```python
from build123d import *

# Parameters (mm, degrees)
RESSALTO_EXTRUS_O1_DEPTH = 4
FILETE1_R                = 3
M3_CLEARANCE_HOLE1_D     = 3.2
FURO_COM_FOLGA_DE_M32_D  = 2.87
M3_CLEARANCE_HOLE2_D     = 3.2
SKETCH3_W                = 27.430623534
SKETCH3_H                = 190
CUT_EXTRUDE1_DEPTH       = 10
BOSS_EXTRUDE1_DEPTH      = 4
FILLET3_R                = 3
BOSS_EXTRUDE3_DEPTH      = 4
M3_CLEARANCE_HOLE4_D     = 3.2
FILLET5_R                = 3
M5_CLEARANCE_HOLE1_D     = 5.3
SKETCH15_R               = 3
CUT_EXTRUDE6_DEPTH       = 5
SKETCH17_W               = 196
SKETCH17_H               = 23.942856981
CUT_EXTRUDE8_DEPTH       = 5
M3_CLEARANCE_HOLE6_D     = 3.2
M3_CLEARANCE_HOLE5_D     = 3.2
CUT_EXTRUDE9_DEPTH       = 4


with BuildPart() as part:
    # Esboço1 → Ressalto-extrusão1 (new body)
    with BuildSketch(Plane.XY):
        with BuildLine():
            Line((168.243612151, -138.115636704), (-79.756387849, -138.115636704))
            ThreePointArc((-79.756387849, -138.115636704), (-80.46349463, -137.822743485), (-80.756387849, -137.115636704))
            Line((-80.756387849, -137.115636704), (-80.756387849, 48.884363296))
            ThreePointArc((-80.756387849, 48.884363296), (-79.877708192, 51.005683639), (-77.756387849, 51.884363296))
            Line((-77.756387849, 51.884363296), (166.243612151, 51.884363296))
            ThreePointArc((166.243612151, 51.884363296), (168.364932495, 51.005683639), (169.243612151, 48.884363296))
            Line((169.243612151, 48.884363296), (169.243612151, -137.115636704))
            ThreePointArc((169.243612151, -137.115636704), (168.950718933, -137.822743485), (168.243612151, -138.115636704))
        make_face()
        with BuildLine():
            Line((-36.756387849, -93.115636704), (-55.756387849, -93.115636704))
            Line((-55.756387849, -93.115636704), (-55.756387849, -79.115636704))
            Line((-55.756387849, -79.115636704), (-55.756387849, 27.884363296))
            ThreePointArc((-55.756387849, 27.884363296), (-54.877708192, 30.005683639), (-52.756387849, 30.884363296))
            Line((-52.756387849, 30.884363296), (141.243612151, 30.884363296))
            ThreePointArc((141.243612151, 30.884363296), (143.364932495, 30.005683639), (144.243612151, 27.884363296))
            Line((144.243612151, 27.884363296), (144.243612151, -79.115636704))
            Line((144.243612151, -79.115636704), (144.243612151, -93.115636704))
            Line((144.243612151, -93.115636704), (125.243612151, -93.115636704))
            Line((125.243612151, -93.115636704), (125.243612151, -107.115636704))
            ThreePointArc((125.243612151, -107.115636704), (124.950718933, -107.822743485), (124.243612151, -108.115636704))
            Line((124.243612151, -108.115636704), (-35.756387849, -108.115636704))
            ThreePointArc((-35.756387849, -108.115636704), (-36.46349463, -107.822743485), (-36.756387849, -107.115636704))
            Line((-36.756387849, -107.115636704), (-36.756387849, -93.115636704))
        make_face(mode=Mode.SUBTRACT)
    extrude(amount=RESSALTO_EXTRUS_O1_DEPTH)

    # Filete1
    filete1_edges = [part.edges().sort_by_distance(p)[0] for p in [
        (-55.756387849, -93.115636704, 2),
        (-36.756387849, -93.115636704, 2),
        (125.243612151, -93.115636704, 2),
        (144.243612151, -93.115636704, 2),
    ]]
    fillet(filete1_edges, radius=FILETE1_R)

    # M3 Clearance Hole1 (through all)
    with Locations(Plane(origin=(0, 0, 0), x_dir=(-1, 0, 0), z_dir=(0, 0, -1))):
        with Locations((-164.230041881, -97.102981335), (43.669958119, -97.102981335), (75.742817578, -97.102981335)):
            Hole(M3_CLEARANCE_HOLE1_D / 2)

    # Furo com folga de M32 (through all)
    with Locations(Plane.XY.offset(4)):
        with Locations((44.243612151, 46.98714614)):
            Hole(FURO_COM_FOLGA_DE_M32_D / 2)

    # M3 Clearance Hole2 (through all)
    with Locations(Plane.XY.offset(4)):
        with Locations((161.560317261, 35.480164232), (161.560317261, 4.480164232)):
            Hole(M3_CLEARANCE_HOLE2_D / 2)

    # Sketch3 → Cut-Extrude1 (cut)
    with BuildSketch(Plane.XY.offset(4)):
        with Locations((169.958923918, -43.115636704)):
            Rectangle(SKETCH3_W, SKETCH3_H)
    extrude(amount=-CUT_EXTRUDE1_DEPTH, mode=Mode.SUBTRACT)

    # Sketch5 → Boss-Extrude1 (add)
    with BuildSketch(Plane(origin=(0, 0, 0), x_dir=(-1, 0, 0), z_dir=(0, 0, -1))):
        with BuildLine():
            Line((-145.240285588, -97.500155699), (-140.243612151, -97.500155699))
            Line((-140.243612151, -97.500155699), (-140.243612151, 27.941506315))
            ThreePointArc((-140.243612151, 27.941506315), (-139.345176524, 30.025791447), (-137.244156422, 30.884363296))
            Line((-137.244156422, 30.884363296), (-145.240285588, 30.884363296))
            Line((-145.240285588, 30.884363296), (-145.240285588, -97.500155699))
        make_face()
    extrude(amount=-BOSS_EXTRUDE1_DEPTH)

    # Fillet3
    fillet3_edges = [part.edges().sort_by_distance(p)[0] for p in [
        (156.243612151, 51.884363296, 2),
    ]]
    fillet(fillet3_edges, radius=FILLET3_R)

    # Sketch10 → Boss-Extrude3 (add)
    with BuildSketch(Plane(origin=(0, 0, 0), x_dir=(-1, 0, 0), z_dir=(0, 0, -1))):
        with BuildLine():
            Line((-156.243612151, -138.115636704), (-156.243612151, 48.884363296))
            ThreePointArc((-156.243612151, 48.884363296), (-155.364932495, 51.005683639), (-153.243612151, 51.884363296))
            Line((-153.243612151, 51.884363296), (-163.743612151, 51.884363296))
            Line((-163.743612151, 51.884363296), (-163.743612151, -138.115636704))
            Line((-163.743612151, -138.115636704), (-156.243612151, -138.115636704))
        make_face()
    extrude(amount=-BOSS_EXTRUDE3_DEPTH)

    # M3 Clearance Hole4 (through all)
    with Locations(Plane(origin=(0, 0, 0), x_dir=(-1, 0, 0), z_dir=(0, 0, -1))):
        with Locations((-160.743612151, -101.615636704), (-160.743612151, -132.615636704), (-129.743612151, -132.615636704), (-129.743612151, -101.615636704)):
            Hole(M3_CLEARANCE_HOLE4_D / 2)

    # Fillet5
    fillet5_edges = [part.edges().sort_by_distance(p)[0] for p in [
        (140.243612151, -93.115636704, 2),
        (163.743612151, 51.884363296, 2),
    ]]
    fillet(fillet5_edges, radius=FILLET5_R)

    # M5 Clearance Hole1 (through all)
    with Locations(Plane(origin=(0, 0, 0), x_dir=(-1, 0, 0), z_dir=(0, 0, -1))):
        with Locations((-115.03361215, -125.8856367), (26.54638785, -125.8856367), (-44.189907873, -129.865636704)):
            Hole(M5_CLEARANCE_HOLE1_D / 2)

    # Sketch15 → Cut-Extrude6 (cut, through all)
    with BuildSketch(Plane(origin=(0, 0, 0), x_dir=(-1, 0, 0), z_dir=(0, 0, -1))):
        with Locations((-145.243612151, -117.115636704)):
            Circle(SKETCH15_R)
    extrude(amount=-CUT_EXTRUDE6_DEPTH, mode=Mode.SUBTRACT)

    # Sketch17 → Cut-Extrude8 (cut)
    with BuildSketch(Plane(origin=(0, 0, 0), x_dir=(-1, 0, 0), z_dir=(0, 0, -1))):
        with Locations((-42.243612151, 39.912934806)):
            Rectangle(SKETCH17_W, SKETCH17_H)
    extrude(amount=-CUT_EXTRUDE8_DEPTH, mode=Mode.SUBTRACT)

    # M3 Clearance Hole6 (through all)
    with Locations(Plane(origin=(0, 0, 0), x_dir=(-1, 0, 0), z_dir=(0, 0, -1))):
        with Locations((-148.743612151, -78.347886704), (-148.743612151, -18.347886704), (-148.743612151, 41.652113296), (60.256387849, 41.652113296), (60.256387849, -18.347886704), (60.256387849, -78.347886704), (72.959751747, -51.945636704)):
            Hole(M3_CLEARANCE_HOLE6_D / 2)

    # M3 Clearance Hole5 (through all)
    with Locations(Plane.XY.offset(4)):
        with Locations((-75.756387849, 41.652113296), (-75.756387849, 48.152113296), (158.743612151, 48.152113296), (158.743612151, 41.652113296)):
            Hole(M3_CLEARANCE_HOLE5_D / 2)

    # Sketch22 → Cut-Extrude9 (cut)
    with BuildSketch(Plane(origin=(0, 0, 0), x_dir=(-1, 0, 0), z_dir=(0, 0, -1))):
        with BuildLine():
            Line((-46.840844325, -129.865636704), (-46.840844325, -123.2156367))
            ThreePointArc((-46.840844325, -123.2156367), (-44.189907873, -120.564700249), (-41.538971422, -123.2156367))
            Line((-41.538971422, -123.2156367), (-41.538971422, -129.865636704))
            ThreePointArc((-41.538971422, -129.865636704), (-44.189907873, -132.516573155), (-46.840844325, -129.865636704))
        make_face()
    extrude(amount=-CUT_EXTRUDE9_DEPTH, mode=Mode.SUBTRACT)


solid = part.part
```
Could you check a few things on this model? Use its own coordinates, in mm. Give positions to 0.01 mm unless a question says otherwise; leave off trailing zeros. Write each loop counter-clockwise with the first axis right and the second up, starting at its lowest first coordinate (ties: lowest second). Pieces come first, ordered by that corner, then holes. Notation, with made-up numbers: (-24, 64.5) -> (-6, 64.5) arc R24 ccw to (-6, 95.5) -> close; hole circle Ø5 at (86, -1.5). An arc over 180 degrees is marked (long way). Write each question's results on one line, items separated by ' | '.
1. I want a section at C-C, the plane x = 50. Write out the boundary of the cut face in (y, z).
Check sheet entries:
outline: (-138.12, 0) -> (-108.12, 0) -> (-108.12, 4) -> (-138.12, 4) -> close
2. Will these pins go through, and if not, where does the flat tip stop? pin 1 Ø1 at (x, z) = (44, 3) entering from +Y; pin 2 Ø1.9 at (x, y) = (129.74, -132.62) entering from -Z.
Check sheet entries:
pin 1: stops at y = -108.12 | pin 2: passes through
3. I want a section at A-A, the plane y = -35.5. Write out the boundary of the cut face in (x, z), then the cut area to 3 significant figures.
Check sheet entries:
outline: (-80.76, 0) -> (-55.76, 0) -> (-55.76, 4) -> (-80.76, 4) -> close; (140.24, 0) -> (163.74, 0) -> (163.74, 4) -> (140.24, 4) -> close | area: 194 mm²
4. If we mould it in two halves opening along Y, with no side actions, what happens to faces 1 (the flat face through (33, -113, 0)), 2 (the cylindrical face through (116.46, -123.65, 2.03))? For each: released by +Y, released by -Y, zero draft, split by the parting line, or undercut.
Check sheet entries:
face 1: zero draft | face 2: undercut
5. I need wall thicknesses on L1, parallel to Y at x = 130, z = 2.55; L2, parallel to X at y = -125.5, z = 1.95; L3, parallel to X at y = -105.5, z = 0.75. Which ranges of each line are inside material? Lowest first, please.
Check sheet entries:
L1: y = -138.12 to -134.19, -131.04 to -103.19, -100.04 to -93.12 | L2: x = -80.76 to -29.17, -23.92 to 41.54, 46.84 to 112.41, 117.66 to 163.74 | L3: x = -80.76 to -36.76, 125.24 to 163.74
6. I want a section at B-B, the plane z = 1.2. Count the separate pieces of the cut face and the enclosed holes in it, then the cut area to 3 significant figures.
Check sheet entries:
separate pieces: 1 | enclosed holes: 21 | area: 15,300 mm²
